For this review, take the finished solid that the model builds, in its own axes (mm). Face numbers are marked on the shaded views. A direction names the side the tool comes from. Round coordinates to 2 decimals unless told otherwise and drop trailing zeros. Write each loop counter-clockwise with the first axis right and the second up, starting at its lowest first coordinate (ties: lowest second). Pieces come first, ordered by that corner, then holes. Notation, with made-up numbers: (11.25, 62.5) -> (30.25, 62.5) arc R29 ccw to (30.25, 87.5) -> close; hole circle Ø7 at (23.5, -25.75). An arc over 180 degrees is marked (long way). Write each question's results on one line, items separated by ' | '. Start each with the question number.
Item 1: Add section C-C (z = -35.5). State the section outline as (x, y) points, plus the area to 3 significant figures.
Item 2: To check wall thickness, follow line 1 along Z through (x, y) = (-13.5, 10.75); line 2 along Z through (x, y) = (42, 21.75); line 3 along X through (y, z) = (15.25, 30.5). State the ranges of each line that lie inside material, in increasing order.
Item 3: Tool access review of the marked faces 4, 5, 6, 7 and 8: name each direction out of +Z, -Z, +X, -X, +Y, -Y from which nothing blocks a thin tool from reaching the whole face with its end or side.
Item 4: Add section B-B (z = 22). State the section outline as (x, y) points.
Item 5: Add section A-A (y = 27.25). State the section outline as (x, z) points, plus the area to 3 significant figures.
Item 6: Clearance check with flat-ended pins moving along their axes: pin 1 (6 mm diameter, centred on x = 0, z = -26, fed in from +Y); pin 2 (4 mm diameter, centred on y = 6.5, z = -28.5, fed in from +X); pin 3 (10 mm diameter, centred on x = 16.5, y = 16.5, fed in from +Z). State where each tip first meets the part, or that it passes through.
Item 7: The part is to be moulded in two halves that separate along Z. For the marked faces 1, 2 and 3, say which applies: +Z half, -Z half, draft (parallel to the pull), parting line (faces both ways), or undercut.
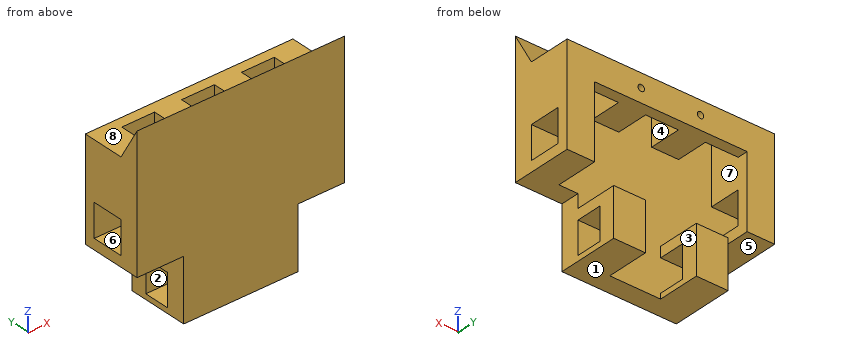
from build123d import *

# Parameters (mm, degrees)
CROQUIS1_W              = 98
CROQUIS1_H              = 98
SALIENTE_EXTRUIR1_DEPTH = 9
CHAFL_N1_SIZE2          = 15.588457268
CHAFL_N1_SIZE           = 9
CROQUIS2_W              = 22
CROQUIS2_H              = 35
CORTAR_EXTRUIR1_DEPTH   = 9
CROQUIS3_W              = 15
CROQUIS3_H              = 2.5
SALIENTE_EXTRUIR2_DEPTH = 12.2
CROQUIS4_W              = 15
CROQUIS4_H              = 20.2
SALIENTE_EXTRUIR3_DEPTH = 2.5
CROQUIS5_W              = 5.9
CROQUIS5_H              = 9
CORTAR_EXTRUIR2_DEPTH   = 54.2
CROQUIS6_W              = 15
CROQUIS6_H              = 14.7
SALIENTE_EXTRUIR4_DEPTH = 2.5
SALIENTE_EXTRUIR5_DEPTH = 20
CROQUIS8_W              = 15.5
CROQUIS8_H              = 15
CORTAR_EXTRUIR3_DEPTH   = 98
CROQUIS9_W              = 15.5
CROQUIS9_H              = 15
CORTAR_EXTRUIR4_DEPTH   = 13
CROQUIS10_W             = 15
CROQUIS10_H             = 22.7
SALIENTE_EXTRUIR6_DEPTH = 5.3
CROQUIS11_R             = 1.5
CORTAR_EXTRUIR5_DEPTH   = 10


with BuildPart() as part:
    # Croquis1 → Saliente-Extruir1 (new body)
    with BuildSketch(Plane(origin=(0, 0, 0), x_dir=(1, 0, 0), z_dir=(0, 1, 0))):
        Rectangle(CROQUIS1_W, CROQUIS1_H)
    extrude(amount=SALIENTE_EXTRUIR1_DEPTH)

    # Chaflán1
    chafl_n1_edges = [part.edges().sort_by_distance(p)[0] for p in [
        (0, 9, 49),
    ]]
    chafl_n1_side = [part.faces().sort_by_distance(p)[0] for p in [
        (0, 8.82, 49),
    ]]
    chamfer(chafl_n1_edges, length=CHAFL_N1_SIZE - 0.0001, length2=CHAFL_N1_SIZE2 - 0.0001, reference=chafl_n1_side[0])  # a hair under: the kernel refuses the full size

    # Croquis2 → Cortar-Extruir1 (cut)
    with BuildSketch(Plane(origin=(0, 9, 0), x_dir=(1, 0, 0), z_dir=(0, 1, 0))):
        with Locations((-38, 31.5)):
            Rectangle(CROQUIS2_W, CROQUIS2_H)
        with Locations((38, 31.5)):
            Rectangle(CROQUIS2_W, CROQUIS2_H)
    extrude(amount=-CORTAR_EXTRUIR1_DEPTH, mode=Mode.SUBTRACT)

    # Croquis3 → Saliente-Extruir2 (add)
    with BuildSketch(Plane(origin=(0, 9, 0), x_dir=(1, 0, 0), z_dir=(0, 1, 0))):
        with Locations((19.5, 41.85)):
            Rectangle(CROQUIS3_W, CROQUIS3_H)
        with Locations((19.5, 24.15)):
            Rectangle(CROQUIS3_W, CROQUIS3_H)
        with Locations((-19.5, 41.85)):
            Rectangle(CROQUIS3_W, CROQUIS3_H)
        with Locations((-19.5, 24.15)):
            Rectangle(CROQUIS3_W, CROQUIS3_H)
    extrude(amount=SALIENTE_EXTRUIR2_DEPTH)

    # Croquis4 → Saliente-Extruir3 (add)
    with BuildSketch(Plane(origin=(0, 21.2, 0), x_dir=(1, 0, 0), z_dir=(0, 1, 0))):
        with Locations((-19.5, 33)):
            Rectangle(CROQUIS4_W, CROQUIS4_H)
        with Locations((19.5, 33)):
            Rectangle(CROQUIS4_W, CROQUIS4_H)
    extrude(amount=SALIENTE_EXTRUIR3_DEPTH)

    # Croquis5 → Cortar-Extruir2 (cut)
    with BuildSketch(Plane(origin=(27, 0, 0), x_dir=(0, 0, -1), z_dir=(1, 0, 0))):
        with Locations((46.05, 4.5)):
            Rectangle(CROQUIS5_W, CROQUIS5_H)
    extrude(amount=-CORTAR_EXTRUIR2_DEPTH, mode=Mode.SUBTRACT)

    # Croquis6 → Saliente-Extruir4 (add)
    with BuildSketch(Plane.XY.offset(-22.9)):
        with Locations((-19.5, 16.35)):
            Rectangle(CROQUIS6_W, CROQUIS6_H)
        with Locations((19.5, 16.35)):
            Rectangle(CROQUIS6_W, CROQUIS6_H)
    extrude(amount=SALIENTE_EXTRUIR4_DEPTH)

    # Croquis7 → Saliente-Extruir5 (add)
    with BuildSketch(Plane(origin=(0, 9, 0), x_dir=(1, 0, 0), z_dir=(0, 1, 0))):
        Polygon((-49, 14), (-49, -33.411542732), (49, -33.411542732), (49, 14), (36, 14), (36, -20.411542732), (-36, -20.411542732), (-36, 14), align=None)
    extrude(amount=SALIENTE_EXTRUIR5_DEPTH)

    # Croquis8 → Cortar-Extruir3 (cut)
    with BuildSketch(Plane(origin=(49, 0, 0), x_dir=(0, 0, -1), z_dir=(1, 0, 0))):
        with Locations((1.25, 16.5)):
            Rectangle(CROQUIS8_W, CROQUIS8_H)
    extrude(amount=-CORTAR_EXTRUIR3_DEPTH, mode=Mode.SUBTRACT)

    # Croquis9 → Cortar-Extruir4 (cut)
    with BuildSketch(Plane.XY.offset(33.411542732)):
        with Locations((-28.25, 16.5)):
            Rectangle(CROQUIS9_W, CROQUIS9_H)
        with Locations((0, 16.5)):
            Rectangle(CROQUIS9_W, CROQUIS9_H)
        with Locations((28.25, 16.5)):
            Rectangle(CROQUIS9_W, CROQUIS9_H)
    extrude(amount=-CORTAR_EXTRUIR4_DEPTH, mode=Mode.SUBTRACT)

    # Croquis10 → Saliente-Extruir6 (add)
    with BuildSketch(Plane(origin=(0, 23.7, 0), x_dir=(1, 0, 0), z_dir=(0, 1, 0))):
        with Locations((-19.5, 31.75)):
            Rectangle(CROQUIS10_W, CROQUIS10_H)
        with Locations((19.5, 31.75)):
            Rectangle(CROQUIS10_W, CROQUIS10_H)
    extrude(amount=SALIENTE_EXTRUIR6_DEPTH)

    # Croquis11 → Cortar-Extruir5 (cut)
    with BuildSketch(Plane(origin=(0, 29, 0), x_dir=(1, 0, 0), z_dir=(0, 1, 0))):
        with Locations(Location((-14, -26.911542732, 0), (0, 0, 270))):
            Circle(CROQUIS11_R)
        with Locations(Location((14, -26.911542732, 0), (0, 0, 270))):
            Circle(CROQUIS11_R)
    extrude(amount=-CORTAR_EXTRUIR5_DEPTH, mode=Mode.SUBTRACT)


solid = part.part
Responses:
1) outline: (-27, 0) -> (27, 0) -> (27, 9) -> (-27, 9) -> close; (-27, 21.2) -> (-12, 21.2) -> (-12, 29) -> (-27, 29) -> close; (12, 21.2) -> (27, 21.2) -> (27, 29) -> (12, 29) -> close | area: 720 mm^2
2) line 1: z = -43.1 to -40.6, -25.4 to -20.4, 20.41 to 33.41 | line 2: z = -14 to -9, 6.5 to 33.41 | line 3: x = -49 to -36, -20.5 to -7.75, 7.75 to 20.5, 36 to 49
3) face 4: +Z, -Z | face 5: -Z, -X, +Y, -Y | face 6: +X, -X | face 7: -Z | face 8: +Z, +X, -X, +Y
4) outline: (-49, 0) -> (49, 0) -> (49, 29) -> (-49, 29) -> close; hole (-36, 9) -> (-20.5, 9) -> (-20.5, 24) -> (-36, 24) -> close; hole (-7.75, 9) -> (7.75, 9) -> (7.75, 24) -> (-7.75, 24) -> close; hole (20.5, 9) -> (36, 9) -> (36, 24) -> (20.5, 24) -> close
5) outline: (-49, -14) -> (-36, -14) -> (-36, 20.41) -> (36, 20.41) -> (36, -14) -> (49, -14) -> (49, 33.41) -> (-49, 33.41) -> close; (-27, -43.1) -> (-12, -43.1) -> (-12, -20.4) -> (-27, -20.4) -> close; (12, -43.1) -> (27, -43.1) -> (27, -20.4) -> (12, -20.4) -> close; hole circle Ø3 at (-14, 26.91); hole circle Ø3 at (14, 26.91) | area: 2,840 mm^2
6) pin 1: stops at y = 9 | pin 2: stops at x = 27 | pin 3: stops at z = 33.41
7) face 1: -Z half | face 2: undercut | face 3: draft
